from build123d import *

# Parameters (mm, degrees)
SKETCH1_W           = 0.35
SKETCH1_H           = 4.5
BOSS_EXTRUDE1_DEPTH = 4.5


with BuildPart() as part:
    # Sketch1 → Boss-Extrude1 (new body)
    with BuildSketch(Plane(origin=(0, 0, 0), x_dir=(1, 0, 0), z_dir=(0, 1, 0))):
        with BuildLine():
            Line((-112.624700466, 140.964918284), (-67.062250697, 140.964918284))
            Line((-67.062250697, 140.964918284), (-67.062250697, 138.264918284))
            Line((-67.062250697, 138.264918284), (-34.817903115, 138.264918284))
            Line((-34.817903115, 138.264918284), (-34.817903115, 140.964918284))
            Line((-34.817903115, 140.964918284), (10.744546655, 140.964918284))
            Line((10.744546655, 140.964918284), (10.744546655, 138.264918284))
            Line((10.744546655, 138.264918284), (20.744546655, 138.264918284))
            Line((20.744546655, 138.264918284), (20.744546655, 138.400653035))
            ThreePointArc((20.744546655, 138.400653035), (23.738342853, 134.832785659), (20.744546655, 131.264918284))
            Line((20.744546655, 131.264918284), (-2.381937072, 127.187095234))
            Line((-2.381937072, 127.187095234), (-3.076529782, 131.126326246))
            Line((-3.076529782, 131.126326246), (-7.508164671, 130.344909446))
            Line((-7.508164671, 130.344909446), (-6.81357196, 126.405678434))
            Line((-6.81357196, 126.405678434), (-45.647003133, 119.558296765))
            Line((-45.647003133, 119.558296765), (-46.341595844, 123.497527777))
            Line((-46.341595844, 123.497527777), (-50.773230733, 122.716110978))
            Line((-50.773230733, 122.716110978), (-50.078638022, 118.776879966))
            Line((-50.078638022, 118.776879966), (-95.69726199, 110.733085737))
            Line((-95.69726199, 110.733085737), (-96.3918547, 114.672316749))
            Line((-96.3918547, 114.672316749), (-100.823489589, 113.89089995))
            Line((-100.823489589, 113.89089995), (-100.128896878, 109.951668938))
            Line((-100.128896878, 109.951668938), (-116.756459578, 107.01978101))
            ThreePointArc((-116.756459578, 107.01978101), (-120.838638515, 108.11359756), (-122.624700466, 111.943819775))
            Line((-122.624700466, 111.943819775), (-122.624700466, 121.171097677))
            Line((-122.624700466, 121.171097677), (-118.624700466, 121.171097677))
            Line((-118.624700466, 121.171097677), (-118.624700466, 125.671097677))
            Line((-118.624700466, 125.671097677), (-122.624700466, 125.671097677))
            Line((-122.624700466, 125.671097677), (-122.624700466, 138.264918284))
            Line((-122.624700466, 138.264918284), (-112.624700466, 138.264918284))
            Line((-112.624700466, 138.264918284), (-112.624700466, 140.964918284))
        make_face()
        Polygon((-3.510650226, 133.588345628), (-7.942285115, 132.806928829), (-8.003061977, 133.151611543), (-3.571427089, 133.933028342), align=None, mode=Mode.SUBTRACT)
        Polygon((-46.775716288, 125.95954716), (-51.207351177, 125.17813036), (-51.268128039, 125.522813074), (-46.83649315, 126.304229873), align=None, mode=Mode.SUBTRACT)
        Polygon((-96.791107352, 117.140484264), (-101.257610033, 116.352919332), (-101.318386895, 116.697602046), (-96.851884214, 117.485166978), align=None, mode=Mode.SUBTRACT)
        with Locations((-115.949700466, 123.421097677)):
            Rectangle(SKETCH1_W, SKETCH1_H, mode=Mode.SUBTRACT)
    extrude(amount=BOSS_EXTRUDE1_DEPTH)


solid = part.part
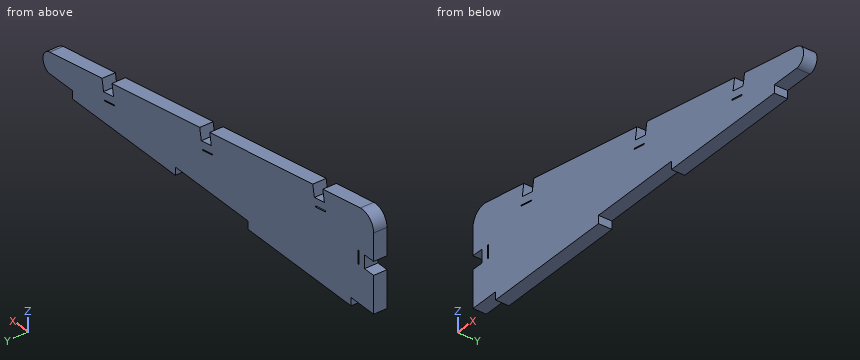
Verification items for the finished model (mm, model axes). Give positions to 0.01 mm unless a question says otherwise; leave off trailing zeros. Loops run counter-clockwise (first coordinate to the right, second up) from the corner with the lowest first, then second, coordinate; pieces in that order, holes last. Notation, with made-up numbers: (7.25, -3) - (26.25, -3) arc R11 ccw to (26.25, 16) - close; hole circle Ø11 at (-28, -33). An arc over 180 degrees is marked (long way). Write each question's results on one line, items separated by ' | '.
1) Depth check by flat-ended pin: P1, Ø0.8, axis at y = 3.5, z = -140.5, coming from the +X side; P2, Ø1.2, axis at x = -120.5, y = 3.5, coming from the -Z side; P3, Ø2, axis at x = -120, y = 2, coming from the +Z side; P4, Ø10, axis at x = -69, z = -115.5, coming from the -Y side. Enter the tip coordinate at first touch or a pass-through.
Solution:
P1: x = 10.74 | P2: z = -138.26 | P3: z = -107.14 | P4: y = 0
2) Sectioned sample at A-A on y = 1.75. Count the separate pieces of the cut face and the enclosed holes in it, plus the area to 3 significant figures.
Solution:
separate pieces: 1 | enclosed holes: 4 | area: 2,990 mm2
3) Sectioned sample at C-C on x = -59. Record the boundary of the cut face in (y, z), plus the area to 3 significant figures.
Solution:
outline: (0, -138.26) - (4.5, -138.26) - (4.5, -117.2) - (0, -117.2) - close | area: 94.8 mm2
4) Sectioned sample at B-B on x = 15. Record the boundary of the cut face in (y, z).
Solution:
outline: (0, -138.26) - (4.5, -138.26) - (4.5, -130.25) - (0, -130.25) - close
5) Material ranges on L1, parallel to X at y = 3.85, z = -140; L2, parallel to Z at x = -85, y = 2.3; L3, parallel to X at y = 1.5, z = -138, recorded low to high. Write a range as from..to.
Solution:
L1: -112.62..-67.06, -34.82..10.74 | L2: -140.96..-112.62 | L3: -122.62..21.87
